```python
from build123d import *

# Parameters (mm, degrees)
F1_DEPTH = 70
F0_R     = 9
F2_DEPTH = 73
F0_R_2   = 10
F3_DEPTH = 15
F0_R_3   = 5
F4_DEPTH = 17
F5_SIZE2 = 9
F5_SIZE  = 9


with BuildPart() as f1:
    # F0 (on Front) → F1 (new body)
    with BuildSketch(Plane.XZ):
        with BuildLine():
            Line((0, 15), (0, 0))
            Line((0, 0), (90, 0))
            Line((90, 0), (90, 15))
            Line((90, 15), (62.860571, 15))
            ThreePointArc((62.860571, 15), (45, 4), (27.139429, 15))
            Line((27.139429, 15), (0, 15))
        make_face()
    extrude(amount=F1_DEPTH)

    # F0 (on Front) → F2 (join)
    with BuildSketch(Plane.XZ):
        with BuildLine():
            ThreePointArc((65, 24), (40.374604, 43.457793), (27.139429, 15))
            ThreePointArc((27.139429, 15), (45, 4), (62.860571, 15))
            ThreePointArc((62.860571, 15), (64.457793, 19.374604), (65, 24))
        make_face()
        with Locations((45, 24)):
            Circle(F0_R, mode=Mode.SUBTRACT)
    extrude(amount=F2_DEPTH)

    # F0 (on Front) → F3 (join)
    with BuildSketch(Plane.XZ):
        with BuildLine():
            Line((0, 70), (0, 15))
            Line((0, 15), (27.139429, 15))
            ThreePointArc((27.139429, 15), (40.374604, 43.457793), (65, 24))
            ThreePointArc((65, 24), (64.457793, 19.374604), (62.860571, 15))
            Line((62.860571, 15), (90, 15))
            Line((90, 15), (90, 70))
            Line((90, 70), (0, 70))
        make_face()
        with Locations((45, 58)):
            Circle(F0_R_2, mode=Mode.SUBTRACT)
    extrude(amount=F3_DEPTH)

    # F0 (on Front) → F4 (join)
    with BuildSketch(Plane.XZ):
        with Locations((45, 58)):
            Circle(F0_R_2)
        with Locations((45, 58)):
            Circle(F0_R_3, mode=Mode.SUBTRACT)
    extrude(amount=F4_DEPTH)

    # F5
    f5_edges = [f1.edges().sort_by_distance(p)[0] for p in [
        (0, -7.5, 70),
        (90, -7.5, 70),
    ]]
    chamfer(f5_edges, length=F5_SIZE, length2=F5_SIZE2)


solid = f1.part
```
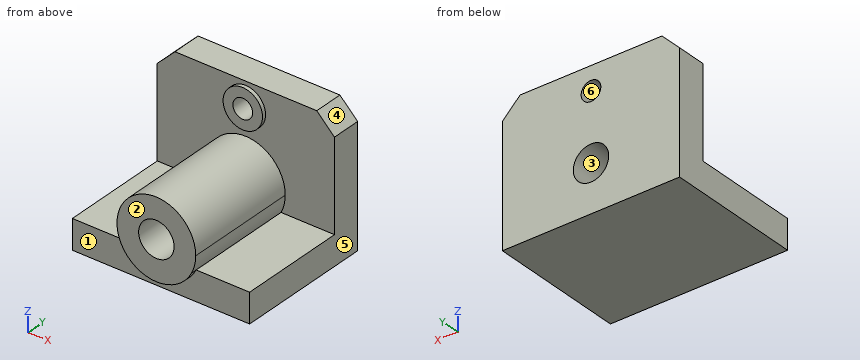
The model under review builds one solid part; all positions refer to its coordinate system, in mm. Face numbers are marked on the shaded views. A direction names the side the tool comes from. Round coordinates to 2 decimals unless told otherwise and drop trailing zeros. Loops run counter-clockwise (first coordinate to the right, second up) from the corner with the lowest first, then second, coordinate; pieces in that order, holes last. Notation, with made-up numbers: (55, -19) - (66, -19) arc R22 cw to (66, 15) - close; hole circle Ø2 at (45.25, 29.25). An arc over 180 degrees is marked (long way). Write each question's results on one line, items separated by ' | '. Start each with the question number.
Q1. Insertion check: P1, Ø8, axis at y = -41, z = 31, coming from the -X side; P2, Ø16, axis at x = 40.5, z = 62.5, coming from the -Y side. Each pin has a flat end and moves straight along its axis. Give the tip position at first contact, or say it passes through.
Q2. Draft analysis for pull direction Z (two halves, no side actions). For the marked faces 3, 4, 5 and 6, state which applies: pulls with the +Z half, pulls with the -Z half, needs draft (parallel to the pull), parting line crosses it, or undercut.
Q3. Tool access review of the marked faces 1 and 2: name each direction out of +Z, -Z, +X, -X, +Y, -Y from which nothing blocks a thin tool from reaching the whole face with its end or side.
Q4. Take a section at D-D on z = 30.5. Give the boundary of the cut face in (x, y).
Q5. Take a section at B-B on x = 45. Give the boundary of the cut face in (y, z), plus the area to 3 significant figures.
Q6. Take a section at C-C on y = -21. Give the boundary of the cut face in (x, z).
Q7. Wall thickness on line 1 along Z through (x, y) = (45, -5.5); line 2 along Z through (x, y) = (45, -55.5); line 3 along Z through (x, y) = (6, -15.5): over which ranges is each line inside the solid? List them lowest first. Write a range as [from, to].
Q8. Take a section at A-A on y = -10. Give the boundary of the cut face in (x, z), plus the area to 3 significant figures.
Data:
1) P1: stops at x = 25.23 | P2: stops at y = -17
2) face 3: undercut | face 4: pulls with the +Z half | face 5: needs draft | face 6: undercut
3) face 1: -Z, -Y | face 2: +Z, -Z, +X, -X, -Y
4) outline: (0, -15) - (26.09, -15) - (26.09, -73) - (38.78, -73) - (38.78, 0) - (0, 0) - close; (51.22, -73) - (63.91, -73) - (63.91, -15) - (90, -15) - (90, 0) - (51.22, 0) - close
5) outline: (-73, 4) - (-70, 4) - (-70, 0) - (0, 0) - (0, 15) - (-73, 15) - close; (-73, 33) - (0, 33) - (0, 53) - (-17, 53) - (-17, 48) - (-15, 48) - (-15, 44) - (-73, 44) - close; (-17, 63) - (0, 63) - (0, 70) - (-15, 70) - (-15, 68) - (-17, 68) - close | area: 2,150 mm²
6) outline: (0, 0) - (90, 0) - (90, 15) - (62.86, 15) arc R20 ccw to (65, 24) arc R20 ccw (long way) to (27.14, 15) - (0, 15) - close; hole circle Ø18 at (45, 24)
7) line 1: z = [0, 15], [33, 53], [63, 70] | line 2: z = [0, 15], [33, 44] | line 3: z = [0, 15]
8) outline: (0, 0) - (90, 0) - (90, 61) - (81, 70) - (9, 70) - (0, 61) - close; hole circle Ø18 at (45, 24); hole circle Ø10 at (45, 58) | area: 5,890 mm²
